Autodesk Inventor part; units mm, degrees
ref_plane "YZ Plane" through (0, 0, 0) normal (1, 0, 0) x (0, 1, 0)
ref_plane "XZ Plane" through (0, 0, 0) normal (0, 1, 0) x (-1, 0, 0)
ref_plane "XY Plane" through (0, 0, 0) normal (0, 0, 1) x (1, 0, 0)
sketch "Sketch1" plane through (0, 0, 0) normal (0, 1, 0) x (-1, 0, 0)
  line L0 (0, 0) -> (-15, 0)
  line L1 (-15, 0) -> (-15, -15)
  line L2 (-15, -15) -> (0, -15)
  line L3 (0, -15) -> (0, 0)
extrude "Plate1" add sketch "Sketch1" along normal blind 1
sketch "Sketch2" plane through (1, 0, 0) normal (-1, 0, 0) x (0, -1, 0)
  line L0 (0, -15) -> (0, 0)
  line L1 (0, 0) -> (-17, 0)
  line L2 (-17, 0) -> (-17, -15)
  line L3 (-17, -15) -> (0, -15)
edge flange "Flange1" height 17 angle 90 thickness 1 bend radius 1 thickness toward (-1, 0, 0) relief tear relief width 1 relief depth 0.5 edges at (0, 1, -7.5) wall of the first edge with corners at (1, 0, -15) (1, 0, 0) (1, 17, 0) (1, 17, -15)
bend "Bend1"
corner "Corner1"
sketch "Sketch3" plane through (0, 1, 0) normal (0, 1, 0) x (1, 0, 0)
  circle A0 centre (13.1306, 13.1131) radius 1
  line L0 (2, 15) -> (15, 15)
  circle A1 centre (13.1306, 1.887) radius 1
  point P0 (0, 0)
extrude "Extrusion1" cut sketch "Sketch3" against normal through all
sketch "Sketch4" plane through (1, 17, 0) normal (1, 0, 0) x (0, 0, -1)
  circle A0 centre (2.6622, -2.6905) radius 1
  circle A1 centre (12.8576, -2.6905) radius 1
  point P0 (0, -17)
extrude "Extrusion2" cut sketch "Sketch4" against normal blind 10
equation "\"d2\" = Thickness"
equation "\"d3\" = BendReliefWidth"
equation "\"d4\" = BendReliefDepth"
equation "\"d5\" = MinimumRemnant"
equation "\"d6\" = TransitionRadius"
equation "\"d9\" = BendRadius"
equation "\"d10\" = CornerReliefSize"
equation "\"d11\" = GapSize"
equation "\"d12\" = JacobiRadiusSize"
equation "\"BendRadius\" = Thickness"
equation "\"BendReliefWidth\" = Thickness"
equation "\"BendReliefDepth\" = 0.5 * Thickness"
equation "\"CornerReliefSize\" = 4 * Thickness"
equation "\"MinimumRemnant\" = 2 * Thickness"
equation "\"TransitionRadius\" = BendRadius"
equation "\"JacobiRadiusSize\" = BendRadius"
equation "\"GapSize\" = Thickness"
properties part number "Clamps"
Could you check a few things on this model? Use its own coordinates, in mm. A direction names the side the tool comes from. Give positions to 0.01 mm unless a question says otherwise; leave off trailing zeros. Order: outer loops, then holes, each group sorted by start corner. A loop starts at its lowest first (then second) coordinate and runs counter-clockwise, first axis right, second up.
Q1. Suppose I cut it at C-C, the plane y = 14.75. Write out the boundary of the cut face in (x, z).
Q2. Suppose I cut it at A-A, the plane x = 13.75. Write out the boundary of the cut face in (y, z).
Q3. If I drill on line 1 along Y through (x, z) = (14.25, -11); line 2 along Y through (x, z) = (1.5, -5.5), over which ranges is the centre line in solid material (lowest first)?
Q4. Suppose I cut it at D-D, the plane z = -10.5. Write out the boundary of the cut face in (x, y), and give its area (3 significant figures).
Q5. Suppose I cut it at B-B, the plane z = -12.75. Write out the boundary of the cut face in (x, y), and give its area (3 significant figures).
Q6. For faces 4 (the flat face through (0, 10, -7)), 5 (the flat face through (1, 9, -7)), which set-ups out of +Z, -Z, +X, -X, +Y, -Y let a thin tool reach every point of the face, with its end or its side?
Q7. We'd pull the mould along Z, two halves only. Please class faces 1 (the flat face through (15, 0.5, -7.4)), 2 (the flat face through (0.8, 4.8, -15)), 3 (the cylindrical face through (14.054, 0.507, -1.504)): +Z half, -Z half, draft (parallel to the pull), parting line (faces both ways), or undercut.
Q8. I'm going to push flat-ended pins straight in: P1, Ø2, axis at y = 10.5, z = -13, coming from the +X side; P2, Ø3, axis at y = 3, z = -5.5, coming from the +X side. Where does each tip first touch, or does it pass through?
Solution:
1. outline: (0, -15) - (1, -15) - (1, -13.76) - (0, -13.76) - close; (0, -11.96) - (1, -11.96) - (1, -3.56) - (0, -3.56) - close; (0, -1.76) - (1, -1.76) - (1, 0) - (0, 0) - close
2. outline: (0, -15) - (1, -15) - (1, -13.9) - (0, -13.9) - close; (0, -12.33) - (1, -12.33) - (1, -2.67) - (0, -2.67) - close; (0, -1.1) - (1, -1.1) - (1, 0) - (0, 0) - close
3. line 1: y = 0 to 1
3. line 2: y = 0.06 to 1.13
4. outline: (0, 2) arc R2 ccw to (2, 0) - (15, 0) - (15, 1) - (2, 1) arc R1 cw to (1, 2) - (1, 17) - (0, 17) - close
4. area: 30.4 mm2
5. outline: (0, 2) arc R2 ccw to (2, 0) - (12.2, 0) - (12.2, 1) - (2, 1) arc R1 cw to (1, 2) - (1, 13.32) - (0, 13.32) - close; (0, 15.3) - (1, 15.3) - (1, 17) - (0, 17) - close; (14.06, 0) - (15, 0) - (15, 1) - (14.06, 1) - close
5. area: 26.5 mm2
6. face 4: +Z, -Z, -X, +Y, -Y
6. face 5: +Z, -Z, +X, +Y
7. face 1: draft
7. face 2: -Z half
7. face 3: undercut
8. P1: stops at x = 1
8. P2: stops at x = 1.13
